The drawing under review shows one solid part. Ordinate dimensions are in mm from its lowest x, y, z. Give positions to 0.01 mm unless a question says otherwise; leave off trailing zeros. Write each loop counter-clockwise with the first axis right and the second up, starting at its lowest first coordinate (ties: lowest second). Pieces come first, ordered by that corner, then holes. Notation, with made-up numbers: (10.25, -4.75) -> (20.25, -4.75) arc R19 ccw to (20.25, 3.25) -> close; hole circle Ø8 at (66, -8.5). An arc over 180 degrees is marked (long way). Use CSV: the item, a comma, the result in double quotes.
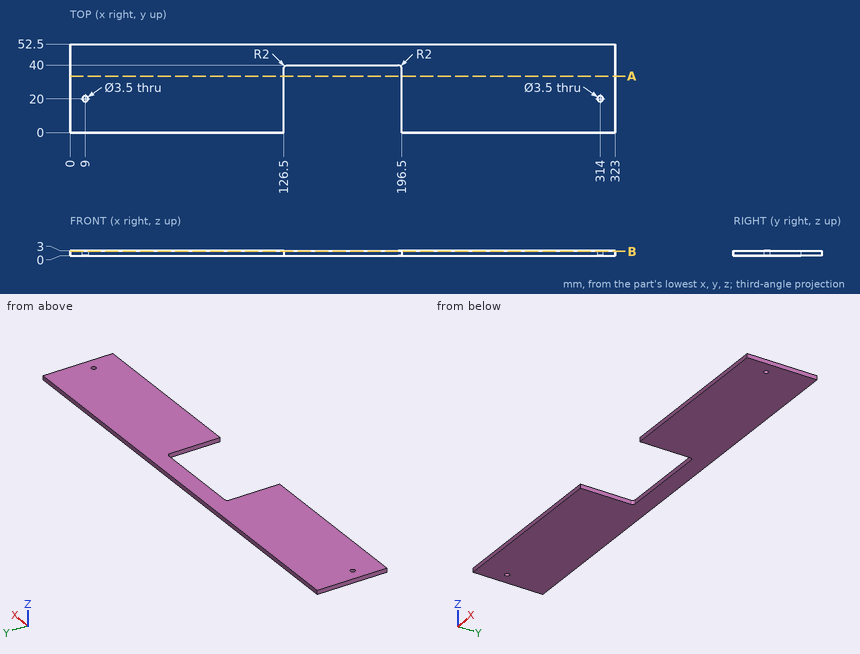
(1) Clearance check with a flat-ended pin moving along its axis: pin 1 (0.9 mm diameter, centred on x = 171.5, z = 2, fed in from -Y). State where the tip first meets the part, or that it passes through.
Established:
pin 1,"stops at y = 40"
(2) Take a section at B-B (z = 2.55). Write out the cut boundary in (x, y), then the cut area to 3 significant figures.
Established:
outline,"(0, 0) -> (126.5, 0) -> (126.5, 38) arc R2 cw to (128.5, 40) -> (194.5, 40) arc R2 cw to (196.5, 38) -> (196.5, 0) -> (323, 0) -> (323, 52.5) -> (0, 52.5) -> close; hole circle Ø3.5 at (9, 20); hole circle Ø3.5 at (314, 20)"
area,"14,100 mm2"
(3) For line 1 along X through (y, z) = (30, 1.1); line 2 along Y through (x, z) = (9, 2.2); line 3 along Y through (x, z) = (177, 0.45), list the stretches that pass through material, from the lowest coordinate up. Write a range as [from, to].
Established:
line 1,"x = [0, 126.5], [196.5, 323]"
line 2,"y = [0, 18.25], [21.75, 52.5]"
line 3,"y = [40, 52.5]"
(4) Take a section at A-A (y = 33.5). Write out the cut boundary in (x, z).
Established:
outline,"(0, 0) -> (126.5, 0) -> (126.5, 3) -> (0, 3) -> close; (196.5, 0) -> (323, 0) -> (323, 3) -> (196.5, 3) -> close"
